from build123d import *

# Parameters (mm, degrees)
F0_R     = 31.75
F1_DEPTH = 0.508
F2_R     = 3.81
F3_DEPTH = 33.02
F4_R     = 3.81
F5_DEPTH = 1.27
F6_R     = 3.81
F7_DEPTH = 2.54


with BuildPart() as f1:
    # F0 (on Top) → F1 (new body)
    with BuildSketch(Plane.XY):
        Circle(F0_R)
    extrude(amount=F1_DEPTH)

    # F2 (on face) → F3 (join)
    with BuildSketch(Plane(origin=(0, 0, 0), x_dir=(1, 0, 0), z_dir=(0, 0, -1))):
        Circle(F2_R)
    extrude(amount=F3_DEPTH)

    # F4 (on face) → F5 (join)
    with BuildSketch(Plane(origin=(0, 0, -33.02), x_dir=(1, 0, 0), z_dir=(0, 0, -1))):
        with BuildLine():
            ThreePointArc((8.255, -3.2995567884), (8.7298066989, -1.6800520825), (8.89, 0))
            ThreePointArc((8.89, 0), (8.7298066989, 1.6800520825), (8.255, 3.2995567884))
            ThreePointArc((8.255, 3.2995567884), (7.6989658396, 4.445), (6.985, 5.499261314))
            ThreePointArc((6.985, 5.499261314), (4.445, 7.6989658396), (1.27, 8.7988181024))
            ThreePointArc((1.27, 8.7988181024), (0, 8.89), (-1.27, 8.7988181024))
            ThreePointArc((-1.27, 8.7988181024), (-4.445, 7.6989658396), (-6.985, 5.499261314))
            ThreePointArc((-6.985, 5.499261314), (-7.6989658396, 4.445), (-8.255, 3.2995567884))
            ThreePointArc((-8.255, 3.2995567884), (-8.89, 0), (-8.255, -3.2995567884))
            ThreePointArc((-8.255, -3.2995567884), (-7.6989658396, -4.445), (-6.985, -5.499261314))
            ThreePointArc((-6.985, -5.499261314), (-4.445, -7.6989658396), (-1.27, -8.7988181024))
            ThreePointArc((-1.27, -8.7988181024), (0, -8.89), (1.27, -8.7988181024))
            ThreePointArc((1.27, -8.7988181024), (4.445, -7.6989658396), (6.985, -5.499261314))
            ThreePointArc((6.985, -5.499261314), (7.6989658396, -4.445), (8.255, -3.2995567884))
        make_face()
        Circle(F4_R, mode=Mode.SUBTRACT)
        Circle(F4_R)
        with BuildLine():
            ThreePointArc((-1.27, 8.7988181024), (0, 8.89), (1.27, 8.7988181024))
            Line((1.27, 8.7988181024), (1.27, 11.3388181024))
            Line((1.27, 11.3388181024), (-1.27, 11.3388181024))
            Line((-1.27, 11.3388181024), (-1.27, 8.7988181024))
        make_face()
        with BuildLine():
            ThreePointArc((6.985, 5.499261314), (7.6989658396, 4.445), (8.255, 3.2995567884))
            Line((8.255, 3.2995567884), (10.4547045256, 4.5695567884))
            Line((10.4547045256, 4.5695567884), (9.1847045256, 6.769261314))
            Line((9.1847045256, 6.769261314), (6.985, 5.499261314))
        make_face()
        with BuildLine():
            Line((10.4547045256, -4.5695567884), (8.255, -3.2995567884))
            ThreePointArc((8.255, -3.2995567884), (7.6989658396, -4.445), (6.985, -5.499261314))
            Line((6.985, -5.499261314), (9.1847045256, -6.769261314))
            Line((9.1847045256, -6.769261314), (10.4547045256, -4.5695567884))
        make_face()
        with BuildLine():
            Line((1.27, -11.3388181024), (1.27, -8.7988181024))
            ThreePointArc((1.27, -8.7988181024), (0, -8.89), (-1.27, -8.7988181024))
            Line((-1.27, -8.7988181024), (-1.27, -11.3388181024))
            Line((-1.27, -11.3388181024), (1.27, -11.3388181024))
        make_face()
        with BuildLine():
            Line((-9.1847045256, -6.769261314), (-6.985, -5.499261314))
            ThreePointArc((-6.985, -5.499261314), (-7.6989658396, -4.445), (-8.255, -3.2995567884))
            Line((-8.255, -3.2995567884), (-10.4547045256, -4.5695567884))
            Line((-10.4547045256, -4.5695567884), (-9.1847045256, -6.769261314))
        make_face()
        with BuildLine():
            ThreePointArc((-8.255, 3.2995567884), (-7.6989658396, 4.445), (-6.985, 5.499261314))
            Line((-6.985, 5.499261314), (-9.1847045256, 6.769261314))
            Line((-9.1847045256, 6.769261314), (-10.4547045256, 4.5695567884))
            Line((-10.4547045256, 4.5695567884), (-8.255, 3.2995567884))
        make_face()
    extrude(amount=F5_DEPTH)

    # F6 (on face) → F7 (join)
    with BuildSketch(Plane(origin=(0, 0, -34.29), x_dir=(1, 0, 0), z_dir=(0, 0, -1))):
        Circle(F6_R)
    extrude(amount=F7_DEPTH)


solid = f1.part
Input: part model. Units: mm. Frame: model coordinates. A direction names the side the tool comes from. Give positions to 0.01 mm unless a question says otherwise; leave off trailing zeros. Order: outer loops, then holes, each group sorted by start corner. A loop starts at its lowest first (then second) coordinate and runs counter-clockwise, first axis right, second up.
Q1. Contact query for flat-ended pins moving along their axis: pin 1 Ø8 at (x, z) = (-9, -11) entering from +Y; pin 2 Ø12 at (x, y) = (-2, -10) entering from -Z; pin 3 Ø1.5 at (y, z) = (-3.5, -8) entering from -X; pin 4 Ø1 at (y, z) = (10.5, -34) entering from -X. Output: stop coordinate, or through.
Checked values:
pin 1: passes through
pin 2: stops at z = -34.29
pin 3: stops at x = -2.64
pin 4: stops at x = -1.27
Q2. Set-up query: faces 1 (the cylindrical face through (-0.83, 3.72, -35.54)), 2 (the cylindrical face through (-4.404, -7.723, -33.646)), 3 (the cylindrical face through (-4.486, 7.675, -33.646)). Return all of +Z, -Z, +X, -X, +Y, -Y with unobstructed straight access to the full face (end or side cutting, diameter ignored); none if empty.
Checked values:
face 1: -Z
face 2: -Z, -Y
face 3: -Z, +Y
Q3. Section C-C on y = -1. Output: boundary loops of the cut face in (x, z).
Checked values:
outline: (-31.73, 0) - (-3.68, 0) - (-3.68, -33.02) - (-8.83, -33.02) - (-8.83, -34.29) - (-3.68, -34.29) - (-3.68, -36.83) - (3.68, -36.83) - (3.68, -34.29) - (8.83, -34.29) - (8.83, -33.02) - (3.68, -33.02) - (3.68, 0) - (31.73, 0) - (31.73, 0.51) - (-31.73, 0.51) - close
Q4. Section A-A on x = 0. Output: boundary loops of the cut face in (y, z), and give its area (3 significant figures).
Checked values:
outline: (-31.75, 0) - (-3.81, 0) - (-3.81, -33.02) - (-11.34, -33.02) - (-11.34, -34.29) - (-3.81, -34.29) - (-3.81, -36.83) - (3.81, -36.83) - (3.81, -34.29) - (11.34, -34.29) - (11.34, -33.02) - (3.81, -33.02) - (3.81, 0) - (31.75, 0) - (31.75, 0.51) - (-31.75, 0.51) - close
area: 332 mm2
Q5. Draft query along X for faces 4 (the cylindrical face through (4.404, 7.723, -33.646)), 5 (the flat face through (0, 5, -34.29)), 6 (the cylindrical face through (-0.83, 3.72, -16.28)). Return one class per face: +X half, -X half, draft (parallel to the pull), parting line (faces both ways), or undercut.
Checked values:
face 4: undercut
face 5: draft
face 6: parting line
Q6. Section B-B on z = -21. Output: boundary loops of the cut face in (x, y), and give its area (3 significant figures).
Checked values:
outline: circle Ø7.62 at (0, 0)
area: 45.6 mm2
Q7. Section D-D on y = 12.5. Output: boundary loops of the cut face in (x, z).
Checked values:
outline: (-29.19, 0) - (29.19, 0) - (29.19, 0.51) - (-29.19, 0.51) - close
Q8. Ray query, probe 1 along Z at (x, y) = (-8, -4.5); probe 2 along Z at (x, y) = (-19.5, 21); probe 3 along X at (y, z) = (2, -9). Return the intervals inside material, ascending.
Checked values:
probe 1: z = -34.29 to -33.02, 0 to 0.51
probe 2: z = 0 to 0.51
probe 3: x = -3.24 to 3.24
